```python
from build123d import *

# Parameters (mm, degrees)
BOSS_EXTRUDE3_DEPTH  = 6.5
SKETCH5_W            = 6.5
SKETCH5_H            = 5.25
BOSS_EXTRUDE4_DEPTH  = 19.65
SKETCH7_W            = 6.5
SKETCH7_H            = 1.65
BOSS_EXTRUDE5_DEPTH  = 1.65
CUT_EXTRUDE1_DEPTH   = 25.96938125
SKETCH10_R           = 1.5
BOSS_EXTRUDE6_DEPTH  = 2.8
FILLET5_R            = 0.5
BOSS_EXTRUDE7_START  = 2.8
BOSS_EXTRUDE7_DEPTH  = 2.8
CUT_EXTRUDE5_DEPTH   = 27.20157438
CUT_EXTRUDE13_DEPTH  = 0.7
SKETCH23_R           = 1.9
CUT_EXTRUDE14_DEPTH  = 27.427684348
SKETCH20_R           = 2.102432725
CUT_EXTRUDE15_DEPTH  = 0.7
SKETCH24_R           = 1.9
CUT_EXTRUDE16_DEPTH  = 27.427684348
SHELL3_START         = -6.9
SHELL3_DEPTH         = 4.25
SHELL3_2_DEPTH       = 3.55
SHELL3_START_2       = 1
SHELL3_3_DEPTH       = 4.5
SHELL3_START_3       = -1.8
SHELL3_4_OUTLINE_R   = 0.5
SHELL3_4_DEPTH       = 10.1
CUT_EXTRUDE21_DEPTH  = 1
SKETCH27_W           = 6.5
SKETCH27_H           = 4.25
BOSS_EXTRUDE8_DEPTH  = 4.3
SKETCH30_R           = 1.182465124
BOSS_EXTRUDE9_DEPTH  = 2.8
FILLET7_R            = 0.5
SKETCH32_R           = 1.225
BOSS_EXTRUDE11_DEPTH = 2.8
FILLET8_R            = 0.5
SKETCH35_W           = 4.5
SKETCH35_H           = 3.3
CUT_EXTRUDE22_DEPTH  = 3.5


with BuildPart() as part:
    # Sketch4 → Boss-Extrude3 (new body)
    with BuildSketch(Plane(origin=(0, 0, 0), x_dir=(0, 0, -1), z_dir=(1, 0, 0))):
        Polygon((3.25, 6.5), (3.05, -1.497710452), (-2.152769119, -6.9), (-3.45, -6.9), (-3.45, 6.5), align=None)
    extrude(amount=BOSS_EXTRUDE3_DEPTH)

    # Sketch5 → Boss-Extrude4 (add)
    with BuildSketch(Plane.XY.offset(3.45)):
        with Locations((3.25, -4.275)):
            Rectangle(SKETCH5_W, SKETCH5_H)
    extrude(amount=BOSS_EXTRUDE4_DEPTH)

    # Sketch7 → Boss-Extrude5 (add)
    with BuildSketch(Plane.XY.offset(3.45)):
        with Locations((3.25, -0.825)):
            Rectangle(SKETCH7_W, SKETCH7_H)
    extrude(amount=BOSS_EXTRUDE5_DEPTH)

    # Sketch8 → Cut-Extrude1 (cut, through all)
    with BuildSketch(Plane(origin=(6.5, 0, 0), x_dir=(0, 0, -1), z_dir=(1, 0, 0))):
        Polygon((-3.45, 0), (-5.1, -1.65), (-5.1, 0), align=None)
    extrude(amount=-CUT_EXTRUDE1_DEPTH, mode=Mode.SUBTRACT)

    # Sketch10 → Boss-Extrude6 (add)
    with BuildSketch(Plane(origin=(6.5, 0, 0), x_dir=(0, 0, -1), z_dir=(1, 0, 0))):
        with Locations((0, 2)):
            Circle(SKETCH10_R)
    extrude(amount=BOSS_EXTRUDE6_DEPTH)

    # Fillet5
    fillet5_edges = [part.edges().sort_by_distance(p)[0] for p in [
        (9.3, 2, 1.5),
    ]]
    fillet(fillet5_edges, radius=FILLET5_R)

    # Sketch13 → Boss-Extrude7 (add)
    with BuildSketch(Plane.ZY.offset(BOSS_EXTRUDE7_START)):
        with BuildLine():
            ThreePointArc((-1.5, 2), (-1.060660172, 0.939339828), (0, 0.5))
            Line((0, 0.5), (0, 2))
            Line((0, 2), (-1.5, 2))
        make_face()
        with BuildLine():
            Line((0, 2), (0, 0.5))
            ThreePointArc((0, 0.5), (1.060660172, 0.939339828), (1.5, 2))
            Line((1.5, 2), (0, 2))
        make_face()
        with BuildLine():
            Line((-1.5, 2), (0, 2))
            Line((0, 2), (0, 3.5))
            ThreePointArc((0, 3.5), (-1.060660172, 3.060660172), (-1.5, 2))
        make_face()
        with BuildLine():
            Line((0, 3.5), (0, 2))
            Line((0, 2), (1.5, 2))
            ThreePointArc((1.5, 2), (1.060660172, 3.060660172), (0, 3.5))
        make_face()
    extrude(amount=-BOSS_EXTRUDE7_DEPTH)

    # Fillet6: read off the stored shape, not the designer's step
    # Fillet6 outline → Fillet6 (revolve, cut)
    with BuildSketch(Plane(origin=(0, 2, 0), x_dir=(0, 1, 0), z_dir=(0, 0, -1))):
        with BuildLine():
            Line((1.5, -2.8), (1.5, -2.3))
            ThreePointArc((1.5, -2.3), (1.353553391, -2.653553391), (1, -2.8))
            Line((1, -2.8), (1.5, -2.8))
        make_face()
    revolve(axis=Axis((0, 2, 0), (1, 0, 0)), mode=Mode.SUBTRACT)

    # Sketch15 → Cut-Extrude5 (cut, through all)
    with BuildSketch(Plane(origin=(0, -1.65, 0), x_dir=(1, 0, 0), z_dir=(0, 1, 0))):
        with BuildLine():
            Line((0, -23.1), (3.25, -23.1))
            ThreePointArc((3.25, -23.1), (1.137389056, -22.336939099), (0, -20.4))
            Line((0, -20.4), (0, -23.1))
        make_face()
        with BuildLine():
            Line((6.5, -23.1), (6.5, -20.4))
            ThreePointArc((6.5, -20.4), (5.362610944, -22.336939099), (3.25, -23.1))
            Line((3.25, -23.1), (6.5, -23.1))
        make_face()
    extrude(amount=-CUT_EXTRUDE5_DEPTH, mode=Mode.SUBTRACT)

    # Sketch16 → Cut-Extrude13 (cut)
    with BuildSketch(Plane(origin=(0, -1.65, 0), x_dir=(1, 0, 0), z_dir=(0, 1, 0))):
        with BuildLine():
            ThreePointArc((3.25, -18.5), (1.15, -20.6), (3.25, -22.7))
            Line((3.25, -22.7), (3.25, -18.5))
        make_face()
        with BuildLine():
            Line((3.25, -18.5), (3.25, -22.7))
            ThreePointArc((3.25, -22.7), (4.73492424, -22.08492424), (5.35, -20.6))
            ThreePointArc((5.35, -20.6), (4.73492424, -19.11507576), (3.25, -18.5))
        make_face()
    extrude(amount=-CUT_EXTRUDE13_DEPTH, mode=Mode.SUBTRACT)

    # Sketch23 → Cut-Extrude14 (cut, through all)
    with BuildSketch(Plane(origin=(0, -2.35, 0), x_dir=(1, 0, 0), z_dir=(0, 1, 0))):
        with Locations(Location((3.25, -20.6, 0), (0, 0, 270))):
            Circle(SKETCH23_R)
    extrude(amount=-CUT_EXTRUDE14_DEPTH, mode=Mode.SUBTRACT)

    # Sketch20 → Cut-Extrude15 (cut)
    with BuildSketch(Plane(origin=(0, -1.65, 0), x_dir=(1, 0, 0), z_dir=(0, 1, 0))):
        with Locations(Location((3.25, -13.797567275, 0), (0, 0, 270))):
            Circle(SKETCH20_R)
    extrude(amount=-CUT_EXTRUDE15_DEPTH, mode=Mode.SUBTRACT)

    # Sketch24 → Cut-Extrude16 (cut, through all)
    with BuildSketch(Plane(origin=(0, -2.35, 0), x_dir=(1, 0, 0), z_dir=(0, 1, 0))):
        with Locations(Location((3.25, -13.797567275, 0), (0, 0, 270))):
            Circle(SKETCH24_R)
    extrude(amount=-CUT_EXTRUDE16_DEPTH, mode=Mode.SUBTRACT)

    # Shell3: read off the stored shape, not the designer's step
    # Shell3 outline → Shell3 (cut)
    with BuildSketch(Plane(origin=(0, 0, 0), x_dir=(1, 0, 0), z_dir=(0, 1, 0)).offset(SHELL3_START)):
        with BuildLine():
            ThreePointArc((1, -11.661545549), (3.25, -10.69513455), (5.5, -11.661545549))
            Line((5.5, -11.661545549), (5.5, -2.45))
            Line((5.5, -2.45), (1, -2.45))
            Line((1, -2.45), (1, -11.661545549))
        make_face()
        with BuildLine():
            ThreePointArc((5.5, -15.933589001), (3.25, -16.9), (1, -15.933589001))
            Line((1, -15.933589001), (1, -18.467513189))
            ThreePointArc((1, -18.467513189), (3.25, -17.5), (5.5, -18.467513189))
            Line((5.5, -18.467513189), (5.5, -15.933589001))
        make_face()
    extrude(amount=SHELL3_DEPTH, mode=Mode.SUBTRACT)

    # Shell3 2 outline → Shell3 2 (cut)
    with BuildSketch(Plane(origin=(0, 0, 0), x_dir=(1, 0, 0), z_dir=(0, 1, 0)).offset(SHELL3_START)):
        with BuildLine():
            ThreePointArc((1, -11.967949829), (3.25, -10.897567275), (5.5, -11.967949829))
            Line((5.5, -11.967949829), (5.5, -11.661545549))
            ThreePointArc((5.5, -11.661545549), (3.25, -10.69513455), (1, -11.661545549))
            Line((1, -11.661545549), (1, -11.967949829))
        make_face()
        with BuildLine():
            ThreePointArc((5.5, -15.627184721), (3.25, -16.697567275), (1, -15.627184721))
            Line((1, -15.627184721), (1, -15.933589001))
            ThreePointArc((1, -15.933589001), (3.25, -16.9), (5.5, -15.933589001))
            Line((5.5, -15.933589001), (5.5, -15.627184721))
        make_face()
        with BuildLine():
            ThreePointArc((5.5, -18.467513189), (3.25, -17.5), (1, -18.467513189))
            Line((1, -18.467513189), (1, -18.770382554))
            ThreePointArc((1, -18.770382554), (3.25, -17.7), (5.5, -18.770382554))
            Line((5.5, -18.770382554), (5.5, -18.467513189))
        make_face()
    extrude(amount=SHELL3_2_DEPTH, mode=Mode.SUBTRACT)

    # Shell3 3 outline → Shell3 3 (cut)
    with BuildSketch(Plane.YZ.offset(SHELL3_START_2)):
        Polygon((-0.414213562, 2.45), (-2.65, 4.685786438), (-2.65, 2.45), (-6.9, 2.45), (-6.9, 2.152769119), (-2.564073304, -2.023020667), (5.5, -2.224680213), (5.5, 2.45), align=None)
    extrude(amount=SHELL3_3_DEPTH, mode=Mode.SUBTRACT)

    # Shell3 4 outline → Shell3 4 (cut)
    with BuildSketch(Plane.YZ.offset(SHELL3_START_3)):
        with Locations((2, 0)):
            Circle(SHELL3_4_OUTLINE_R)
    extrude(amount=SHELL3_4_DEPTH, mode=Mode.SUBTRACT)

    # Sketch25 → Cut-Extrude21 (cut)
    with BuildSketch(Plane(origin=(0, 6.5, 0), x_dir=(1, 0, 0), z_dir=(0, 1, 0))):
        Polygon((0.853996383, 0.275), (2.051998191, -1.8), (4.448001809, -1.8), (5.646003617, 0.275), (4.448001809, 2.35), (2.051998191, 2.35), align=None)
    extrude(amount=-CUT_EXTRUDE21_DEPTH, mode=Mode.SUBTRACT)

    # Sketch27 → Boss-Extrude8 (add)
    with BuildSketch(Plane(origin=(0, -0.077160181, -3.085523923), x_dir=(-1, 0, 0), z_dir=(0, -0.02499934134114434, -0.9996874676280127))):
        with Locations((-3.25, 2.154216399)):
            Rectangle(SKETCH27_W, SKETCH27_H)
    extrude(amount=BOSS_EXTRUDE8_DEPTH)

    # Sketch30 → Boss-Extrude9 (add)
    with BuildSketch(Plane(origin=(6.5, 0, 0), x_dir=(0, 0, -1), z_dir=(1, 0, 0))):
        with Locations((5.937940908, 1.983914598)):
            Circle(SKETCH30_R)
    extrude(amount=BOSS_EXTRUDE9_DEPTH)

    # Fillet7
    fillet7_edges = [part.edges().sort_by_distance(p)[0] for p in [
        (9.3, 1.983914598, -4.755475784),
    ]]
    fillet(fillet7_edges, radius=FILLET7_R)

    # Sketch32 → Boss-Extrude11 (add)
    with BuildSketch(Plane.ZY):
        with Locations(Location((-5.938343158, 2, 0), (0, 0, 180))):
            Circle(SKETCH32_R)
    extrude(amount=BOSS_EXTRUDE11_DEPTH)

    # Fillet8
    fillet8_edges = [part.edges().sort_by_distance(p)[0] for p in [
        (-2.8, 2, -4.713343158),
    ]]
    fillet(fillet8_edges, radius=FILLET8_R)

    # Sketch35 → Cut-Extrude22 (cut)
    with BuildSketch(Plane(origin=(0, 0.029207268, -0.000730391), x_dir=(1, 0, 0), z_dir=(0, -0.9996874676280127, 0.024999341341144354))):
        with Locations((3.25, -4.736488551)):
            Rectangle(SKETCH35_W, SKETCH35_H)
    extrude(amount=-CUT_EXTRUDE22_DEPTH, mode=Mode.SUBTRACT)


solid = part.part
```
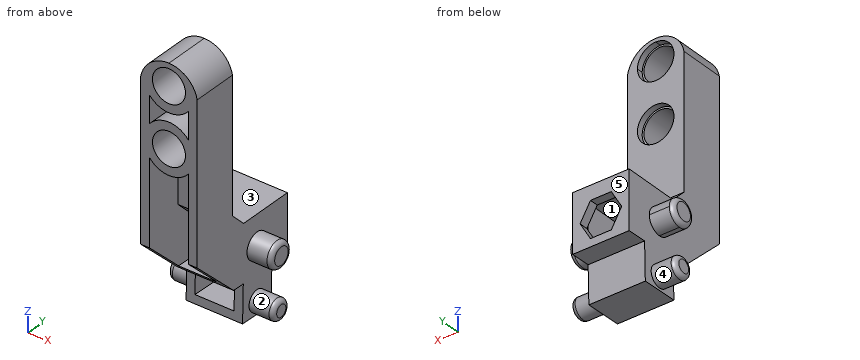
Source: CAD feature listing. Evaluate the final solid. Frame: model axes, mm. Face numbers are marked on the shaded views. A direction names the side the tool comes from. Coordinates: 2 decimals unless noted, no trailing zeros. Write each loop counter-clockwise with the first axis right and the second up, starting at its lowest first coordinate (ties: lowest second). Pieces come first, ordered by that corner, then holes. Notation, with made-up numbers: M -12.75,83 L 8.25,83 A24 cw 8.25,111 Z; hole C 36,31.5 d6. An arc over 180 degrees is marked long. Answer as a JSON object with one key per item and string values.
1. Cut plane A-A on x = -0.5. Output: boundary loops of the cut face in (y, z) (3 decimals), plus the area to 3 significant figures.
Evaluation:
{"outline": "C 2,0 d3; C 2,-5.938 d2.45; hole C 2,0 d1", "area": "11.0 mm^2"}
2. Cut plane B-B on z = 14. Output: boundary loops of the cut face in (x, y), plus the area to 3 significant figures.
Evaluation:
{"outline": "M 0,-6.9 L 1.36,-6.9 L 1.36,-2.35 L 1.16,-2.35 L 1.16,-1.65 L 0,-1.65 Z; M 5.14,-6.9 L 6.5,-6.9 L 6.5,-1.65 L 5.34,-1.65 L 5.34,-2.35 L 5.14,-2.35 Z", "area": "14.0 mm^2"}
3. Access query for the marked faces 1, 2, 3, 4 and 5. Directions: +Z, -Z, +X, -X, +Y, -Y. A direction counts if a zero-diameter tool reaches every point of the face in a straight line with its end or side. Return the directions, or none.
Evaluation:
{"face 1": "-Y", "face 2": "+X", "face 3": "+Z, +X, -X, +Y", "face 4": "-X", "face 5": "+Z, -Z, +X, -X, +Y"}
4. Contact query for flat-ended pins moving along their axis: P1, Ø4.5, axis at x = 2.5, z = 20.5, coming from the +Y side; P2, Ø6.5, axis at y = 0.5, z = 9, coming from the -X side; P3, Ø0.5, axis at x = 3.5, y = 6, coming from the -Z side. Output: stop coordinate, or through.
Evaluation:
{"P1": "y = -1.65", "P2": "x = 0", "P3": "z = -3.24"}
5. Cut plane D-D on x = 2.75. State how many separate pieces and enclosed holes the cut face has, plus the area to 3 significant figures.
Evaluation:
{"separate pieces": "4", "enclosed holes": "0", "area": "51.7 mm^2"}
6. Ray query, L1, parallel to Z at x = -0.8, y = 2; L2, parallel to X at y = -4.25, z = 6.5; L3, parallel to Y at x = -0.05, z = 0. Return the intervals inside material, ascending.
Evaluation:
{"L1": "-7.16 to -4.71, -1.5 to -0.5, 0.5 to 1.5", "L2": "0 to 1, 5.5 to 6.5", "L3": "0.5 to 1.5, 2.5 to 3.5"}
7. Cut plane C-C on y = 5. Output: boundary loops of the cut face in (x, z), plus the area to 3 significant figures.
Evaluation:
{"outline": "M 0,-3.21 L 6.5,-3.21 L 6.5,3.45 L 0,3.45 Z; hole M 1,-2.21 L 5.5,-2.21 L 5.5,2.45 L 1,2.45 Z", "area": "22.3 mm^2"}
